Geometry check sheet. Reference: the model listing, model coordinates, mm. Face numbers are marked on the shaded views. A direction names the side the tool comes from. Coordinates: 2 decimals unless noted, no trailing zeros. Write each loop counter-clockwise with the first axis right and the second up, starting at its lowest first coordinate (ties: lowest second). Pieces come first, ordered by that corner, then holes. Notation, with made-up numbers: M 49,72.25 L 84,72.25 A16 cw 84,77.25 Z; hole C 17.25,3 d1. An arc over 180 degrees is marked long. Write each question's results on one line, items separated by ' | '.
Autodesk Inventor part; units mm, degrees
ref_plane "YZ Plane" through (0, 0, 0) normal (1, 0, 0) x (0, 1, 0)
ref_plane "XZ Plane" through (0, 0, 0) normal (0, 1, 0) x (-1, 0, 0)
ref_plane "XY Plane" through (0, 0, 0) normal (0, 0, 1) x (1, 0, 0)
sketch "Skizze1" plane through (0, 0, 0) normal (0, 0, 1) x (1, 0, 0)
  circle A0 centre (0, 0) radius 12.5
  dimension "d0" = 25
extrude "Extrusion1" add sketch "Skizze1" along normal blind 65
sketch "Skizze2" plane through (0, 0, 65) normal (0, 0, 1) x (1, 0, 0)
  circle A0 centre (0, 0) radius 3.5
  dimension "d3" = 7
extrude "Extrusion2" add sketch "Skizze2" along normal blind 3
sketch "Skizze3" plane through (0, 0, 68) normal (0, 0, 1) x (1, 0, 0)
  arc A0 (1.7321, -1) -> (-1.7321, -1) centre (0, 0) ccw
  line L0 (0, 2) -> (0, -1)
  line L1 (-1.7321, -1) -> (1.7321, -1)
  dimension "d6" = 4
  dimension "d7" = 3
extrude "Extrusion3" add sketch "Skizze3" along normal blind 10
properties part number "Motorskizze"
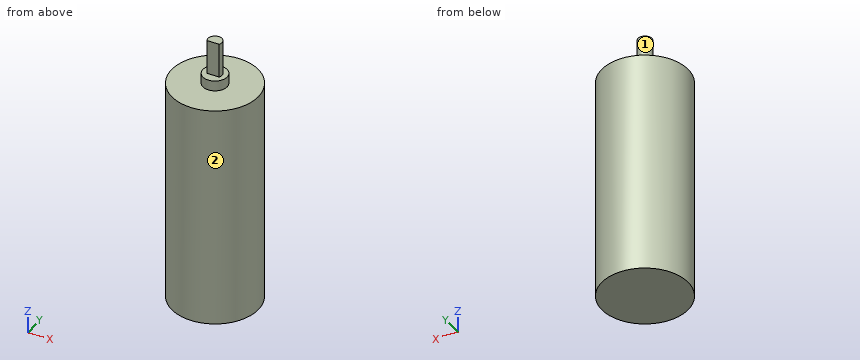
Q1. Sectioned sample at C-C on z = 25.5. Record the cut outline in (x, y).
Geometry check:
outline: C 0,0 d25
Q2. Scan lines: probe 1 along Z at (x, y) = (-7.75, -5); probe 2 along Y at (x, z) = (-0.25, 60.5); probe 3 along Z at (x, y) = (-1, -2.5). Record each from-to range of solid material in increasing order.
Geometry check:
probe 1: z = 0 to 65 | probe 2: y = -12.5 to 12.5 | probe 3: z = 0 to 68
Q3. Sectioned sample at B-B on y = 0. Record the cut outline in (x, z), and give its area (3 significant figures).
Geometry check:
outline: M -12.5,0 L 12.5,0 L 12.5,65 L 3.5,65 L 3.5,68 L 2,68 L 2,78 L -2,78 L -2,68 L -3.5,68 L -3.5,65 L -12.5,65 Z | area: 1,690 mm2
Q4. Access from +Z, -Z, +X, -X, +Y, -Y to the whole of each face (thin tool, end or side, straight path). Record for the marked faces 1 and 2.
Geometry check:
face 1: +Z | face 2: +Z, -Z
Q5. Sectioned sample at D-D on x = -10. Record the cut outline in (y, z), and give its area (3 significant figures).
Geometry check:
outline: M -7.5,0 L 7.5,0 L 7.5,65 L -7.5,65 Z | area: 975 mm2
Q6. Sectioned sample at A-A on x = 0. Record the cut outline in (y, z), and give its area (3 significant figures).
Geometry check:
outline: M -12.5,0 L 12.5,0 L 12.5,65 L 3.5,65 L 3.5,68 L 2,68 L 2,78 L -1,78 L -1,68 L -3.5,68 L -3.5,65 L -12.5,65 Z | area: 1,680 mm2
Q7. Depth check by flat-ended pin: P1, Ø10, axis at x = 6, z = 13, coming from the +Y side; P2, Ø5, axis at y = 8.5, z = 49.5, coming from the +X side; P3, Ø10, axis at x = -8.5, z = 51, coming from the -Y side. Enter the tip coordinate at first touch or a pass-through.
Geometry check:
P1: stops at y = 12.46 | P2: stops at x = 10.97 | P3: stops at y = -12
